Read the model definition and answer for the solid it produces. Units are mm, in the model's axes. Coordinates: 2 decimals unless noted, no trailing zeros. Loops run counter-clockwise (first coordinate to the right, second up) from the corner with the lowest first, then second, coordinate; pieces in that order, holes last.
Q1. Straight lines are drawn through the part: line 1 (Y direction, x = 147.5, z = 3.15); line 2 (Y direction, x = 172, z = 1.7). For each, find the intervals that lie inside material, in ascending order.
Q2. Section A-A (z = 1.8) is taken. Give the vertices of the cut face in (x, y).
Q3. Section B-B (x = 22) is taken. Give the vertices of the cut face in (y, z), then the cut area to 3 significant figures.
from build123d import *

# Parameters (mm, degrees)
BOSS_EXTRU_1_DEPTH = 5


with BuildPart() as part:
    # Esquisse1 → Boss.-Extru.1 (new body)
    with BuildSketch(Plane.XY):
        Polygon((0, 0), (260, 0), (260, 17.454191866), (222.581237858, 24.650107663), (223.053356342, 27.10512378), (223.525474826, 29.560139898), (260, 22.545808134), (260, 90), (0, 90), (0, 72.545808134), (36.474525174, 65.531476369), (36.002406689, 63.076460252), (35.530288205, 60.621444135), (0, 67.454191866), align=None)
        Polygon((72.476931863, 56.062128488), (72.949050347, 58.517144605), (109.423575521, 51.502812841), (108.951457037, 49.047796724), (108.479338552, 46.592780606), (72.004813379, 53.60711237), align=None, mode=Mode.SUBTRACT)
        Polygon((145.42598221, 42.03346496), (145.898100694, 44.488481077), (182.372625868, 37.474149313), (181.900507384, 35.019133195), (181.4283889, 32.564117078), (144.953863726, 39.578448842), align=None, mode=Mode.SUBTRACT)
    extrude(amount=BOSS_EXTRU_1_DEPTH)


solid = part.part
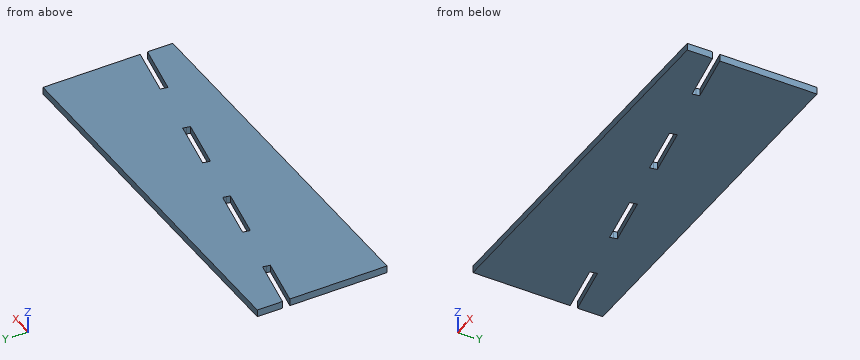
Numbers:
1. line 1: y = 0 to 39.09, 44.18 to 90
1. line 2: y = 0 to 34.38, 39.47 to 90
2. outline: (0, 0) - (260, 0) - (260, 17.45) - (222.58, 24.65) - (223.53, 29.56) - (260, 22.55) - (260, 90) - (0, 90) - (0, 72.55) - (36.47, 65.53) - (35.53, 60.62) - (0, 67.45) - close; hole (72, 53.61) - (108.48, 46.59) - (109.42, 51.5) - (72.95, 58.52) - close; hole (144.95, 39.58) - (181.43, 32.56) - (182.37, 37.47) - (145.9, 44.49) - close
3. outline: (0, 0) - (63.22, 0) - (63.22, 5) - (0, 5) - close; (68.32, 0) - (90, 0) - (90, 5) - (68.32, 5) - close
3. area: 425 mm2
